Could you check a few things on this model? Use its own coordinates, in mm. Face numbers are marked on the shaded views. Coordinates: 2 decimals unless noted, no trailing zeros. Loops run counter-clockwise (first coordinate to the right, second up) from the corner with the lowest first, then second, coordinate; pieces in that order, holes last. Notation, with made-up numbers: (70, -29.75) - (77, -29.75) arc R32 ccw to (77, -2.75) - close; hole circle Ø8 at (87.5, 46.5). An arc over 180 degrees is marked (long way). One line per question, with ' | ' between items. Start each with the question number.
1. Please list where these lines run through material, in increasing order: L1, parallel to X at y = -0.05, z = 0; L2, parallel to X at y = 0.7, z = 20; L3, parallel to X at y = -1.2, z = 2. Write a range as [from, to].
2. I'm going to push flat-ended pins straight in: P1, Ø3.5, axis at x = 20, z = 0, coming from the +Y side; P2, Ø2, axis at y = 0, z = 16, coming from the +X side. Where does each tip first touch, or does it pass through?
3. I want a section at C-C, the plane x = 0. Write out the boundary of the cut face in (y, z).
4. I want a section at A-A, the plane z = 20. Write out the boundary of the cut face in (x, y), then the cut area to 3 significant figures.
5. We'd pull the mould along Z, two halves only. Please class the marked faces 1, 2 and 3: pulls with the +Z half, pulls with the -Z half, needs draft (parallel to the pull), parting line crosses it, or undercut.
6. I want a section at B-B, the plane x = 20. Write out the boundary of the cut face in (y, z).
7. I want a section at D-D, the plane z = 0. Write out the boundary of the cut face in (x, y).
from build123d import *

# Parameters (mm, degrees)
SKETCH1_R           = 2.75
BOSS_EXTRUDE1_DEPTH = 2.3749


with BuildPart() as part:
    # Sketch1 → Boss-Extrude1 (new, symmetric)
    with BuildSketch(Plane(origin=(0, 0, 0), x_dir=(1, 0, 0), z_dir=(0, 1, 0))):
        with BuildLine():
            Line((-10, 7.5), (-10, -27.5))
            ThreePointArc((-10, -27.5), (-9.267766953, -29.267766953), (-7.5, -30))
            Line((-7.5, -30), (7.5, -30))
            ThreePointArc((7.5, -30), (9.267766953, -29.267766953), (10, -27.5))
            Line((10, -27.5), (10, -12.5))
            ThreePointArc((10, -12.5), (10.732233047, -10.732233047), (12.5, -10))
            Line((12.5, -10), (47.5, -10))
            ThreePointArc((47.5, -10), (49.267766953, -9.267766953), (50, -7.5))
            Line((50, -7.5), (50, 7.5))
            ThreePointArc((50, 7.5), (49.267766953, 9.267766953), (47.5, 10))
            Line((47.5, 10), (-7.5, 10))
            ThreePointArc((-7.5, 10), (-9.267766953, 9.267766953), (-10, 7.5))
        make_face()
        with Locations(Location((0, 0, 0), (0, 0, 270))):
            Circle(SKETCH1_R, mode=Mode.SUBTRACT)
        with Locations(Location((20, 0, 0), (0, 0, 270))):
            Circle(SKETCH1_R, mode=Mode.SUBTRACT)
        with Locations(Location((40, 0, 0), (0, 0, 270))):
            Circle(SKETCH1_R, mode=Mode.SUBTRACT)
        with Locations(Location((0, -20, 0), (0, 0, 270))):
            Circle(SKETCH1_R, mode=Mode.SUBTRACT)
    extrude(amount=BOSS_EXTRUDE1_DEPTH, both=True)


solid = part.part
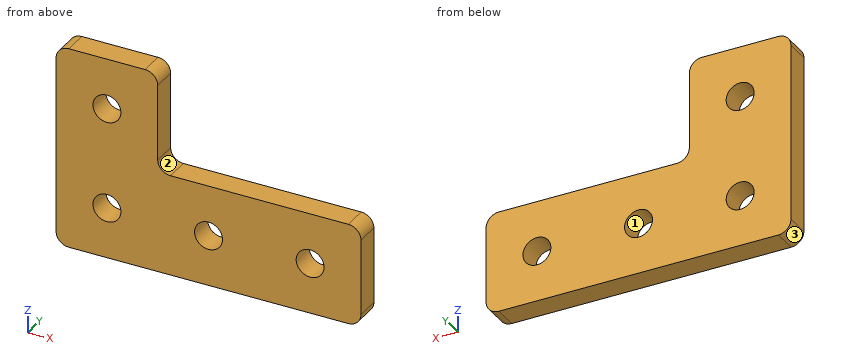
Results are:
1) L1: x = [-10, -2.75], [2.75, 17.25], [22.75, 37.25], [42.75, 50] | L2: x = [-10, -2.75], [2.75, 10] | L3: x = [-10, -1.89], [1.89, 18.11], [21.89, 38.11], [41.89, 50]
2) P1: passes through | P2: stops at x = 10
3) outline: (-2.37, -10) - (2.37, -10) - (2.37, -2.75) - (-2.37, -2.75) - close; (-2.37, 2.75) - (2.37, 2.75) - (2.37, 17.25) - (-2.37, 17.25) - close; (-2.37, 22.75) - (2.37, 22.75) - (2.37, 30) - (-2.37, 30) - close
4) outline: (-10, -2.37) - (-2.75, -2.37) - (-2.75, 2.37) - (-10, 2.37) - close; (2.75, -2.37) - (10, -2.37) - (10, 2.37) - (2.75, 2.37) - close | area: 68.9 mm2
5) face 1: undercut | face 2: pulls with the +Z half | face 3: pulls with the -Z half
6) outline: (-2.37, -10) - (2.37, -10) - (2.37, -2.75) - (-2.37, -2.75) - close; (-2.37, 2.75) - (2.37, 2.75) - (2.37, 10) - (-2.37, 10) - close
7) outline: (-10, -2.37) - (-2.75, -2.37) - (-2.75, 2.37) - (-10, 2.37) - close; (2.75, -2.37) - (17.25, -2.37) - (17.25, 2.37) - (2.75, 2.37) - close; (22.75, -2.37) - (37.25, -2.37) - (37.25, 2.37) - (22.75, 2.37) - close; (42.75, -2.37) - (50, -2.37) - (50, 2.37) - (42.75, 2.37) - close
